Could you check a few things on this model? Use its own coordinates, in mm. A direction names the side the tool comes from. Round coordinates to 2 decimals unless told otherwise and drop trailing zeros. Loops run counter-clockwise (first coordinate to the right, second up) from the corner with the lowest first, then second, coordinate; pieces in that order, holes last. Notation, with made-up numbers: M -3.75,-11.75 L 28.25,-11.75 A18 cw 28.25,20.25 Z; hole C 17.5,67 d9. An arc over 180 degrees is marked long. Answer in a Markdown table with one row per item.
```python
from build123d import *

# Parameters (mm, degrees)
F1_DEPTH = 1


with BuildPart() as f1:
    # F0 (on Front) → F1 (new body, symmetric)
    with BuildSketch(Plane.XZ):
        with BuildLine():
            Line((-150, 300), (-200, 300))
            Line((-200, 300), (-200, -300))
            Line((-200, -300), (-150, -300))
            ThreePointArc((-150, -300), (-135.355339, -264.644661), (-100, -250))
            Line((-100, -250), (100, -250))
            ThreePointArc((100, -250), (135.355339, -264.644661), (150, -300))
            Line((150, -300), (200, -300))
            Line((200, -300), (200, 300))
            Line((200, 300), (150, 300))
            ThreePointArc((150, 300), (135.355339, 264.644661), (100, 250))
            Line((100, 250), (-100, 250))
            ThreePointArc((-100, 250), (-135.355339, 264.644661), (-150, 300))
        make_face()
    extrude(amount=F1_DEPTH, both=True)


solid = f1.part
```
1) If we mould it in two halves opening along X, with no side actions, what happens to faces 4 (the face through (-3, -1, 4)), 5 (the face through (-135.742, -0.014, -265.036)), 6 (the face through (135.742, -0.014, 265.036))? For each: released by +X, released by -X, zero draft, split by the parting line, or undercut.
Computed:
| item | result |
|---|---|
| face 4 | zero draft |
| face 5 | undercut |
| face 6 | undercut |
2) Will these pins go through, and if not, where does the flat tip stop? P1, Ø0.6, axis at x = -26, y = -0.5, coming from the +Z side; P2, Ø1, axis at x = 31, y = -0.5, coming from the -Z side.
Computed:
| item | result |
|---|---|
| P1 | stops at z = 250 |
| P2 | stops at z = -250 |
3) I want a section at B-B, the plane x = -10. Please give me the cut outline in (y, z).
Computed:
| item | result |
|---|---|
| outline | M -1,-250 L 1,-250 L 1,250 L -1,250 Z |
4) I want a section at A-A, the plane y = -0.25. Please give me the cut outline in (x, z).
Computed:
| item | result |
|---|---|
| outline | M -200,-300 L -150,-300 A50 cw -100,-250 L 100,-250 A50 cw 150,-300 L 200,-300 L 200,300 L 150,300 A50 cw 100,250 L -100,250 A50 cw -150,300 L -200,300 Z |
5) I need wall thicknesses on line 1 (Z direction, x = 79.5, y = -0.8); line 2 (X direction, y = -0.1, z = 255); line 3 (Z direction, x = 134.5, y = 0.4). Which ranges of each line are inside material? Lowest first, please.
Computed:
| item | result |
|---|---|
| line 1 | z = -250 to 250 |
| line 2 | x = -200 to -121.79, 121.79 to 200 |
| line 3 | z = -263.81 to 263.81 |
6) Which directions (+Z, -Z, +X, -X, +Y, -Y) give clear straight access to the entire face, cutting with the end or side of a thin tool? Please do faces 1 (the face through (-134.964, -0.014, 264.258)), 2 (the face through (134.964, -0.014, -264.258)), 3 (the face through (-3, 1, 4)).
Computed:
| item | result |
|---|---|
| face 1 | +Z, +Y, -Y |
| face 2 | -Z, +Y, -Y |
| face 3 | +Z, -Z, +X, -X, +Y |
